Check sheet for the modelled part. Datum: model origin and axes. Units: mm. Give positions to 0.01 mm unless a question says otherwise; leave off trailing zeros. Answer in a Markdown table with one row per item. Add a question column.
(1) Go/stop test with flat-tipped pins: P1, Ø0.6, axis at y = -4, z = 88.5, coming from the -X side; P2, Ø0.8, axis at y = -14, z = 132, coming from the +X side; P3, Ø5, axis at x = 0.5, z = 208.5, coming from the -Y side. Record where each tip stops, or that it passes through.
(2) Thickness scan on L1, parallel to Y at x = -12.75, z = 93 (3 decimals); L2, parallel to Y at x = 3.75, z = 97.5. Record the ranges inside material, lowest first.
(3) Sectioned sample at A-A on z = 257.5. State how many separate pieces and enclosed holes the cut face has, then the cut area to 3 significant figures.
from build123d import *

# Parameters (mm, degrees)
BOSS_EXTRUDE1_DEPTH     = 317.5
CUT_EXTRUDE1_DEPTH      = 1
CUT_EXTRUDE1_DEPTH_BACK = 318.5


with BuildPart() as part:
    # Sketch4 → Boss-Extrude1 (new body)
    with BuildSketch(Plane.XY):
        with BuildLine():
            Line((0, -5.45), (0.655464476, -6))
            Line((0.655464476, -6), (4.504469158, -6))
            Line((4.504469158, -6), (8.25, -9.745530842))
            Line((8.25, -9.745530842), (8.25, -12.885))
            Line((8.25, -12.885), (4, -12.885))
            Line((4, -12.885), (4, -14.45))
            Line((4, -14.45), (4.55, -14.45))
            Line((4.55, -14.45), (4.55, -15))
            Line((4.55, -15), (12.885, -15))
            ThreePointArc((12.885, -15), (14.380530842, -14.380530842), (15, -12.885))
            Line((15, -12.885), (15, -4.55))
            Line((15, -4.55), (14.45, -4.55))
            Line((14.45, -4.55), (14.45, -4))
            Line((14.45, -4), (12.885, -4))
            Line((12.885, -4), (12.885, -8.25))
            Line((12.885, -8.25), (9.745530842, -8.25))
            Line((9.745530842, -8.25), (6, -4.504469158))
            Line((6, -4.504469158), (6, -0.655464476))
            Line((6, -0.655464476), (5.45, 0))
            Line((5.45, 0), (3.5, 0))
            ThreePointArc((3.5, 0), (3.371433308, -0.939913534), (2.995178599, -1.81077474))
            Line((2.995178599, -1.81077474), (4.675743591, -3.491339732))
            Line((4.675743591, -3.491339732), (3.491339732, -4.675743591))
            Line((3.491339732, -4.675743591), (1.81077474, -2.995178599))
            ThreePointArc((1.81077474, -2.995178599), (0.939913534, -3.371433308), (0, -3.5))
            Line((0, -3.5), (0, -5.45))
        make_face()
        with BuildLine():
            Line((9.375, -10.365), (9.375, -12.885))
            ThreePointArc((9.375, -12.885), (9.664964287, -13.585035713), (10.365, -13.875))
            Line((10.365, -13.875), (12.885, -13.875))
            ThreePointArc((12.885, -13.875), (13.585035713, -13.585035713), (13.875, -12.885))
            Line((13.875, -12.885), (13.875, -10.365))
            ThreePointArc((13.875, -10.365), (13.585035713, -9.664964287), (12.885, -9.375))
            Line((12.885, -9.375), (10.365, -9.375))
            ThreePointArc((10.365, -9.375), (9.664964287, -9.664964287), (9.375, -10.365))
        make_face(mode=Mode.SUBTRACT)
    extrude(amount=BOSS_EXTRUDE1_DEPTH)

    # Mirror1: part across plane


with BuildPart() as part_1:
    add(part.part)
    add(part.part.mirror(Plane(origin=(0, 0, 0), x_dir=(0, 0, 1), z_dir=(1, 0, 0))))

    # Mirror2: part across plane


with BuildPart() as part_2:
    add(part_1.part)
    add(part_1.part.mirror(Plane.ZX))

    # Sketch5 → Cut-Extrude1 (cut, two sides)
    with BuildSketch(Plane.XY.offset(317.5)) as cut_extrude1_sk:
        Polygon((-5.675, 12.885), (-5.4, 13.16), (-5.125, 12.885), align=None)
    extrude(amount=CUT_EXTRUDE1_DEPTH, mode=Mode.SUBTRACT)
    extrude(cut_extrude1_sk.sketch, amount=-CUT_EXTRUDE1_DEPTH_BACK, mode=Mode.SUBTRACT)


solid = part_2.part
Reply:
| question | item | result |
|---|---|---|
| 1 | P1 | x = -14.45 |
| 1 | P2 | x = 14.88 |
| 1 | P3 | y = -6 |
| 2 | L1 | -15 to -13.875, -9.375 to -8.25, 8.25 to 9.375, 13.875 to 15 |
| 2 | L2 | -6 to -4.42, -2.57 to 2.57, 4.42 to 6 |
| 3 | separate pieces | 1 |
| 3 | enclosed holes | 5 |
| 3 | area | 295 mm^2 |
